The model under review builds one solid part; all positions refer to its coordinate system, in mm. A direction names the side the tool comes from. Round coordinates to 2 decimals unless told otherwise and drop trailing zeros. Loops run counter-clockwise (first coordinate to the right, second up) from the corner with the lowest first, then second, coordinate; pieces in that order, holes last. Notation, with made-up numbers: M 3,39.25 L 55,39.25 A11 cw 55,56.25 Z; hole C -12.75,-8 d3. An arc over 180 degrees is marked long. Use a Markdown table: item, result. Add a question column.
Autodesk Inventor part; units mm, degrees
ref_plane "YZ Plane" through (0, 0, 0) normal (1, 0, 0) x (0, 1, 0)
ref_plane "XZ Plane" through (0, 0, 0) normal (0, 1, 0) x (-1, 0, 0)
ref_plane "XY Plane" through (0, 0, 0) normal (0, 0, 1) x (1, 0, 0)
sketch "Sketch1" plane through (0, 0, 0) normal (0, 1, 0) x (-1, 0, 0)
  line L0 (6, 0) -> (110, 0)
  line L1 (110, 0) -> (110, -104)
  line L2 (104, -110) -> (0, -110)
  line L3 (0, -110) -> (0, -6)
  arc A0 (104, -110) -> (110, -104) centre (104, -104) ccw
  arc A1 (6, 0) -> (0, -6) centre (6, -6) ccw
  point P0 (0, 0)
  point P1 (110, -110)
  dimension "d0" = 110
  dimension "d1" = 110
  dimension "d2" = 6
extrude "Extrusion1" add sketch "Sketch1" along normal blind 3
fillet "Fillet1" radius 6 2 edges at (-110, 1.5, 0) (0, 1.5, -110)
sketch "Sketch3" plane through (0, 0, 0) normal (0, -1, 0) x (1, 0, 0)
  line L0 (-88, -106.5) -> (-96, -106.5)
  line L1 (-96, -106.5) -> (-96, -104)
  line L2 (-96, -104) -> (-88, -104)
  line L3 (-88, -104) -> (-88, -106.5)
  line L4 (-6, -110) -> (-104, -110)
  line L5 (-110, -104) -> (-110, -6)
  line L6 (-14, -106.5) -> (-22, -106.5)
  line L7 (-22, -106.5) -> (-22, -104)
  line L8 (-22, -104) -> (-14, -104)
  line L9 (-14, -104) -> (-14, -106.5)
  line L10 (-88, -6) -> (-96, -6)
  line L11 (-96, -6) -> (-96, -3.5)
  line L12 (-96, -3.5) -> (-88, -3.5)
  line L13 (-88, -3.5) -> (-88, -6)
  line L14 (-14, -6) -> (-22, -6)
  line L15 (-22, -6) -> (-22, -3.5)
  line L16 (-22, -3.5) -> (-14, -3.5)
  line L17 (-14, -3.5) -> (-14, -6)
  line L18 (-106.5, -96) -> (-104, -96)
  line L19 (-104, -96) -> (-104, -88)
  line L20 (-104, -88) -> (-106.5, -88)
  line L21 (-106.5, -88) -> (-106.5, -96)
  line L22 (-106.5, -22) -> (-104, -22)
  line L23 (-104, -14) -> (-106.5, -14)
  line L24 (-104, -22) -> (-104, -14)
  line L25 (-106.5, -14) -> (-106.5, -22)
  line L26 (-6, -96) -> (-3.5, -96)
  line L27 (-3.5, -88) -> (-6, -88)
  line L28 (-3.5, -96) -> (-3.5, -88)
  line L29 (-6, -88) -> (-6, -96)
  line L30 (-6, -22) -> (-3.5, -22)
  line L31 (-3.5, -14) -> (-6, -14)
  line L32 (-3.5, -22) -> (-3.5, -14)
  line L33 (-6, -14) -> (-6, -22)
  point P0 (0, 0)
  dimension "d20" = 8
  dimension "d21" = 2.5
  dimension "d22" = 3.5
  dimension "d23" = 14
  dimension "d26" = 74
  dimension "d29" = 100.5
  dimension "d55" = 8
  dimension "d56" = 2.5
  dimension "d57" = 14
  dimension "d60" = 74
  dimension "d63" = 100.5
  dimension "d66" = 3.5
extrude "Extrusion3" add sketch "Sketch3" along normal blind 8.1
sketch "Sketch4" plane through (-88, 0, -106.5) normal (0, 0, -1) x (-1, 0, 0)
  line L0 (0, 0) -> (0, -8.1)
  line L1 (8, -8.1) -> (0, -8.1)
  line L2 (0, -8.1) -> (0, -4.1)
  line L3 (0, -4.1) -> (8, -4.1)
  line L4 (8, -4.1) -> (8, -8.1)
  line L5 (8, -8.1) -> (0, -8.1)
  line L6 (8, 0) -> (8, -8.1)
  line L7 (-66, 0) -> (-66, -8.1)
  line L8 (-74, 0) -> (-74, -8.1)
  line L9 (-66, -8.1) -> (-74, -8.1)
  line L10 (-74, -8.1) -> (-74, -4.1)
  line L11 (-74, -4.1) -> (-66, -4.1)
  line L12 (-66, -4.1) -> (-66, -8.1)
  point P0 (-88, 0)
  point P1 (0, -8.1)
  dimension "d34" = 4
  dimension "d35" = 0
  dimension "d36" = 0
  dimension "d37" = 4
extrude "Extrusion4" add sketch "Sketch4" along normal blind 2
chamfer "Chamfer1" distance 3 angle 45 2 edges at (-92, -8.1, -108.5) (-18, -8.1, -108.5)
fillet "Fillet2" radius 1 6 edges at (-92, -5.1, -108.5) (-18, -5.1, -108.5) (-18, -8.1, -105.5) (-92, -8.1, -105.5) (-92, -8.1, -104) (-18, -8.1, -104)
fillet "Fillet3" radius 0.5 2 edges at (-92, -4.1, -108.5) (-18, -4.1, -108.5)
sketch "Sketch5" plane through (-96, 0, -3.5) normal (0, 0, 1) x (1, 0, 0)
  line L0 (8, 0) -> (8, -8.1)
  line L1 (0, 0) -> (0, -8.1)
  line L2 (8, -8.1) -> (0, -8.1)
  line L3 (0, -8.1) -> (0, -4.05)
  line L4 (0, -4.05) -> (8, -4.05)
  line L5 (8, -4.05) -> (8, -8.1)
  line L6 (82, -8.1) -> (74, -8.1)
  line L7 (82, -8.1) -> (74, -8.1)
  line L8 (74, -8.1) -> (74, -4.1)
  line L9 (74, -4.1) -> (82, -4.1)
  line L10 (82, -4.1) -> (82, -8.1)
  point P0 (96, 0)
  point P1 (8, -4.05)
  dimension "d45" = 4.05
extrude "Extrusion5" add sketch "Sketch5" along normal blind 2
chamfer "Chamfer2" distance 3 angle 45 2 edges at (-92, -8.1, -1.5) (-18, -8.1, -1.5)
fillet "Fillet4" radius 1 6 edges at (-18, -8.1, -4.5) (-18, -5.1, -1.5) (-18, -8.1, -6) (-92, -8.1, -4.5) (-92, -5.1, -1.5) (-92, -8.1, -6)
fillet "Fillet5" radius 0.5 2 edges at (-92, -4.05, -1.5) (-18, -4.1, -1.5)
fillet "Fillet6" radius 1 1 edges at (-92, 0, -104)
fillet "Fillet7" radius 1 3 edges at (-18, 0, -104) (-18, 0, -6) (-92, 0, -6)
sketch "Sketch6" plane through (0, -8.1, 0) normal (0, -1, 0) x (1, 0, 0)
  line L0 (-104, -96) -> (-106.5, -96)
  line L1 (-104, -88) -> (-104, -96)
  line L2 (-106.5, -96) -> (-104, -96)
  line L3 (-104, -96) -> (-104, -88)
  line L4 (-104, -88) -> (-106.5, -88)
  line L5 (-106.5, -88) -> (-106.5, -96)
  line L6 (-106.5, -22) -> (-106.5, -14)
  line L7 (-106.5, -22) -> (-104, -22)
  line L8 (-104, -22) -> (-104, -14)
  line L9 (-104, -14) -> (-106.5, -14)
  line L10 (-106.5, -14) -> (-106.5, -22)
  line L11 (-6, -14) -> (-6, -22)
  line L12 (-3.5, -22) -> (-3.5, -14)
  line L13 (-6, -22) -> (-3.5, -22)
  line L14 (-3.5, -22) -> (-3.5, -14)
  line L15 (-3.5, -14) -> (-6, -14)
  line L16 (-6, -14) -> (-6, -22)
  line L17 (-3.5, -88) -> (-6, -88)
  line L18 (-6, -88) -> (-6, -96)
  line L19 (-6, -96) -> (-3.5, -96)
  line L20 (-3.5, -96) -> (-3.5, -88)
  point P0 (0, 0)
extrude "Extrusion6" cut sketch "Sketch6" against normal blind 4.5
chamfer "Chamfer3" distance 1 angle 45 4 edges at (-3.5, -3.6, -18) (-3.5, -3.6, -92) (-106.5, -3.6, -92) (-106.5, -3.6, -18)
equation "\"d26\" = d0 - d20 - 2 * d23"
equation "\"d29\" = d1 - d21 - 2 * d22"
equation "\"d55\" = d20"
equation "\"d56\" = d21"
equation "\"d57\" = d23"
equation "\"d60\" = d26"
equation "\"d63\" = d29"
equation "\"d66\" = d22"
properties part number "Cover side-2"
(1) For faces 4 (the face through (-105, -2, -14)), 5 (the face through (-106.5, -1, -92)), 6 (the face through (-104, -2, -92)), list the 3-axis set-ups (+Z, -Z, +X, -X, +Y, -Y) from which the entire face can be reached by the end or side of a thin tool; tool diameter is ignored.
(2) Draft analysis for pull direction Y (two halves, no side actions). For faces 1 (the face through (-18, -4, -104)), 2 (the face through (-92.1, -6.6, -3)), 3 (the face through (-92, -2, -106.5)), state which applies: released by +Y, released by -Y, zero draft, split by the parting line, or undercut.
(3) Consider section A-A, the plane z = -92. Give the boundary of the cut face in (x, y).
(4) To check wall thickness, follow probe 1 along Y at (x, z) = (-43, -36.5); probe 2 along Z at (x, y) = (-16.5, -3.25). State the ranges of each line that lie inside material, in increasing order.
(5) Consider section C-C, the plane z = -29. Give the boundary of the cut face in (x, y), then the cut area to 3 significant figures.
(6) Insertion check: pin 1 Ø1.2 at (x, y) = (-105, -1) entering from -Z; pin 2 Ø1.2 at (x, y) = (-17, -2.5) entering from -Z; pin 3 Ø0.8 at (x, y) = (-5, -2) entering from +Z. Each pin has a flat end and moves straight along its axis. Give the tip position at first contact, or say it passes through.
(7) Consider section B-B, the plane x = -86. Give the boundary of the cut face in (y, z).
Found:
| question | item | result |
|---|---|---|
| 1 | face 4 | +Z, +X, -X, -Y |
| 1 | face 5 | +Z, -Z, -X, -Y |
| 1 | face 6 | +Z, -Z, -Y |
| 2 | face 1 | zero draft |
| 2 | face 2 | released by -Y |
| 2 | face 3 | undercut |
| 3 | outline | M -110,0 L -106.5,0 L -106.5,-2.6 L -105.5,-3.6 L -104,-3.6 L -104,0 L -6,0 L -6,-3.6 L -4.5,-3.6 L -3.5,-2.6 L -3.5,0 L 0,0 L 0,3 L -110,3 Z |
| 4 | probe 1 | y = 0 to 3 |
| 4 | probe 2 | z = -106.5 to -104, -6 to -3.5 |
| 5 | outline | M -110,0 L 0,0 L 0,3 L -110,3 Z |
| 5 | area | 330 mm^2 |
| 6 | pin 1 | stops at z = -96 |
| 6 | pin 2 | stops at z = -106.5 |
| 6 | pin 3 | stops at z = -14 |
| 7 | outline | M 0,-110 L 3,-110 L 3,0 L 0,0 Z |
